from build123d import *

# Parameters (mm, degrees)
F0_W     = 361.95
F0_H     = 247.65
F1_DEPTH = 9.525
F3_D     = 30


# Not quite as in the source:
# - a feature names something its author has since deleted; it is built from what else it names


with BuildPart() as f1:
    # F0 (on Top) → F1 (new body)
    with BuildSketch(Plane.XY):
        with Locations((-148.0553561452, 71.3610090315)):
            Rectangle(F0_W, F0_H)
    extrude(amount=-F1_DEPTH)

    # F3 (through all)
    with Locations(Plane(origin=(0, 0, -9.525), x_dir=(1, 0, 0), z_dir=(0, 0, -1))):
        with Locations((-236.1291795969, -111.6871535778), (-236.1291795969, -156.0809910297), (-198.7664848566, -111.6871535778), (-274.1136550903, -156.0809910297), (-198.7664848566, -156.0809910297), (-274.1136550903, -111.6871535778)):
            Hole(F3_D / 2)


solid = f1.part
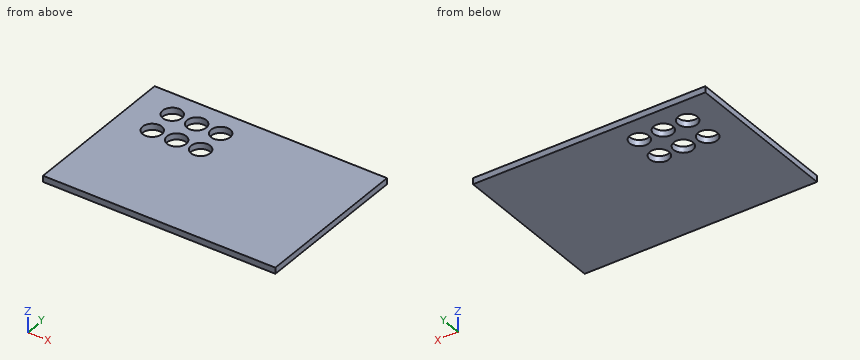
Could you check a few things on this model? Use its own coordinates, in mm. Coordinates: 2 decimals unless noted, no trailing zeros. Write each loop counter-clockwise with the first axis right and the second up, starting at its lowest first coordinate (ties: lowest second). Pieces come first, ordered by that corner, then holes. Notation, with made-up numbers: (57, -13.75) - (100, -13.75) arc R24 cw to (100, 21.25) - close; hole circle Ø2 at (68, 39). An arc over 180 degrees is marked (long way). Write item = value, one per line.
1) Suppose I cut it at B-B on y = 121.5. Please give me the cut outline in (x, z) (3 decimals).
Result set:
outline = (-329.03, -9.525) - (-285.459, -9.525) - (-285.459, 0) - (-329.03, 0) - close; (-262.769, -9.525) - (-247.474, -9.525) - (-247.474, 0) - (-262.769, 0) - close; (-224.784, -9.525) - (-210.111, -9.525) - (-210.111, 0) - (-224.784, 0) - close; (-187.422, -9.525) - (32.92, -9.525) - (32.92, 0) - (-187.422, 0) - close
2) Suppose I cut it at A-A on z = -5.5. Please give me the cut outline in (x, y), plus the area to 3 significant figures.
Result set:
outline = (-329.03, -52.46) - (32.92, -52.46) - (32.92, 195.19) - (-329.03, 195.19) - close; hole circle Ø30 at (-274.11, 111.69); hole circle Ø30 at (-274.11, 156.08); hole circle Ø30 at (-236.13, 111.69); hole circle Ø30 at (-236.13, 156.08); hole circle Ø30 at (-198.77, 111.69); hole circle Ø30 at (-198.77, 156.08)
area = 85,400 mm2
3) Suppose I cut it at C-C on x = -272. Please give me the cut outline in (y, z) (3 decimals).
Result set:
outline = (-52.464, -9.525) - (96.837, -9.525) - (96.837, 0) - (-52.464, 0) - close; (126.537, -9.525) - (141.231, -9.525) - (141.231, 0) - (126.537, 0) - close; (170.931, -9.525) - (195.186, -9.525) - (195.186, 0) - (170.931, 0) - close
4) Will this pin go through, and if not, where does the flat tip stop? pin 1 Ø24 at (x, y) = (-274.11, 156.08) entering from +Z.
Result set:
pin_1 = through
5) Please list where these lines run through material, in increasing order: line 1 (X direction, y = 104.5, z = -0.75); line 2 (X direction, y = 164, z = -6); line 3 (Y direction, x = -234, z = -8.25). Write a range as [from, to].
Result set:
line_1 = [-329.03, -287.28], [-260.95, -249.3], [-222.96, -211.93], [-185.6, 32.92]
line_2 = [-329.03, -286.85], [-261.37, -248.87], [-223.39, -211.51], [-186.03, 32.92]
line_3 = [-52.46, 96.84], [126.54, 141.23], [170.93, 195.19]
